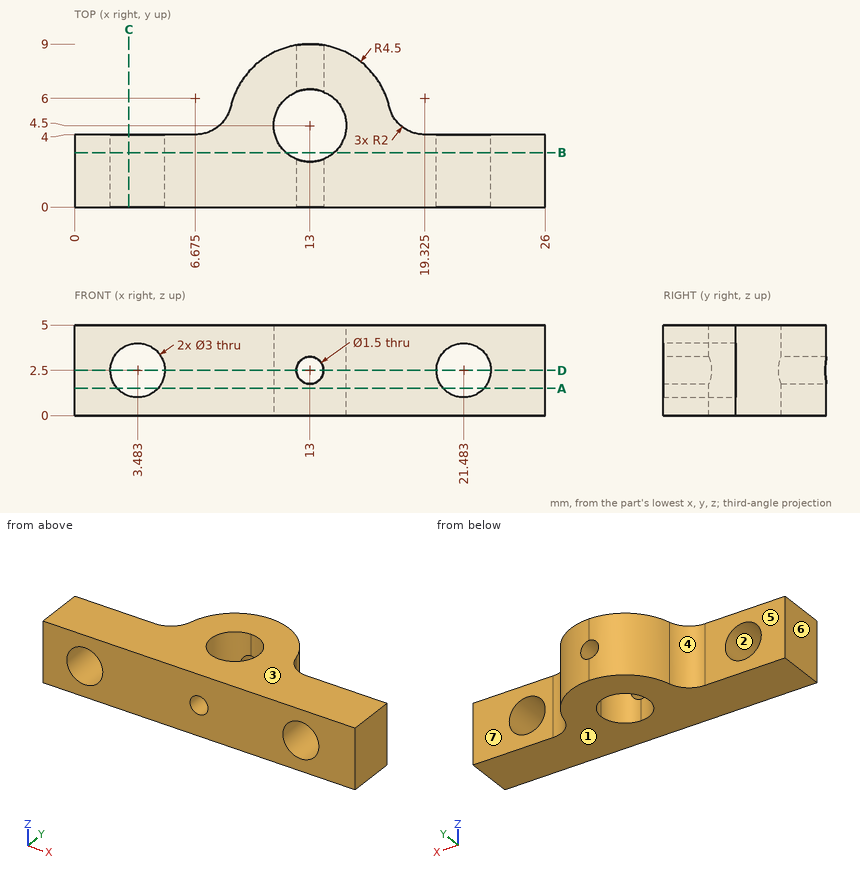
Job drawing, mm, ordinate dimensions from the low corner. One solid piece. A direction names the side the tool comes from. Round coordinates to 2 decimals unless told otherwise and drop trailing zeros. Order: outer loops, then holes, each group sorted by start corner. A loop starts at its lowest first (then second) coordinate and runs counter-clockwise, first axis right, second up. Notation, with made-up numbers: (-37.75, 57.25) - (11.25, 57.25) arc R19 ccw to (11.25, 66.25) - close; hole circle Ø8 at (36.25, 74.25). An arc over 180 degrees is marked (long way). Use CSV: the item, a comma, the result in double quotes. Start each with the question number.
1) Pin check, flat tips, straight feed: pin 1 Ø3 at (x, z) = (6, 3) entering from +Y; pin 2 Ø2.5 at (x, z) = (2.5, 2) entering from +Y. Stop position of each tip, or through.
2) Wall check: L1, parallel to X at y = 1.2, z = 2.5; L2, parallel to Z at x = 13, y = 7.8; L3, parallel to X at y = 0.5, z = 1.4 (1 decimal). Give the ranges that are in metal, low to high. Write a range as [from, to].
3) Saw through at D-D (z = 2.5). Count the separate pieces of the cut face and the enclosed holes in it.
4) Saw through at A-A (z = 1.5). List the corners of the cut face in (x, y) (1 decimal), and give its area (3 significant figures).
5) Two-plate mould, pull along Z, no slides. Class the marked faces 1, 2, 3 and 4: pulls with the +Z half, pulls with the -Z half, needs draft (parallel to the pull), parting line crosses it, or undercut.
6) Saw through at C-C (x = 3). List the corners of the cut face in (y, z).
7) Tool access for the marked faces 5, 6 and 7: list every direction of +Z, -Z, +X, -X, +Y, -Y with a clear straight run to the whole face (end or side of a thin tool).
8) Saw through at B-B (y = 3). List the corners of the cut face in (x, z), and give its area (3 significant figures).
Values follow:
1,pin 1,"stops at y = 4.18"
1,pin 2,"stops at y = 4"
2,L1,"x = [0, 1.98], [4.98, 12.25], [13.75, 19.98], [22.98, 26]"
2,L2,"z = [0, 1.75], [3.25, 5]"
2,L3,"x = [0, 2.5], [4.5, 20.5], [22.5, 26]"
3,separate pieces,"4"
3,enclosed holes,"0"
4,outline,"(0, 0) - (2.4, 0) - (2.4, 4) - (0, 4) - close; (4.6, 0) - (20.4, 0) - (20.4, 4) - (19.3, 4) arc R2 cw to (17.4, 5.5) arc R4.5 ccw to (8.6, 5.5) arc R2 cw to (6.7, 4) - (4.6, 4) - close; (22.6, 0) - (26, 0) - (26, 4) - (22.6, 4) - close; hole circle Ø4 at (13, 4.5)"
4,area,"111 mm2"
5,face 1,"pulls with the -Z half"
5,face 2,"undercut"
5,face 3,"pulls with the +Z half"
5,face 4,"needs draft"
6,outline,"(0, 0) - (4, 0) - (4, 1.08) - (0, 1.08) - close; (0, 3.92) - (4, 3.92) - (4, 5) - (0, 5) - close"
7,face 5,"+Z, -Z, -X, +Y"
7,face 6,"+Z, -Z, -X, +Y, -Y"
7,face 7,"+Z, -Z, +X, +Y"
8,outline,"(0, 0) - (11.68, 0) - (11.68, 5) - (0, 5) - close; (14.32, 0) - (26, 0) - (26, 5) - (14.32, 5) - close; hole circle Ø3 at (3.48, 2.5); hole circle Ø3 at (21.48, 2.5)"
8,area,"103 mm2"
